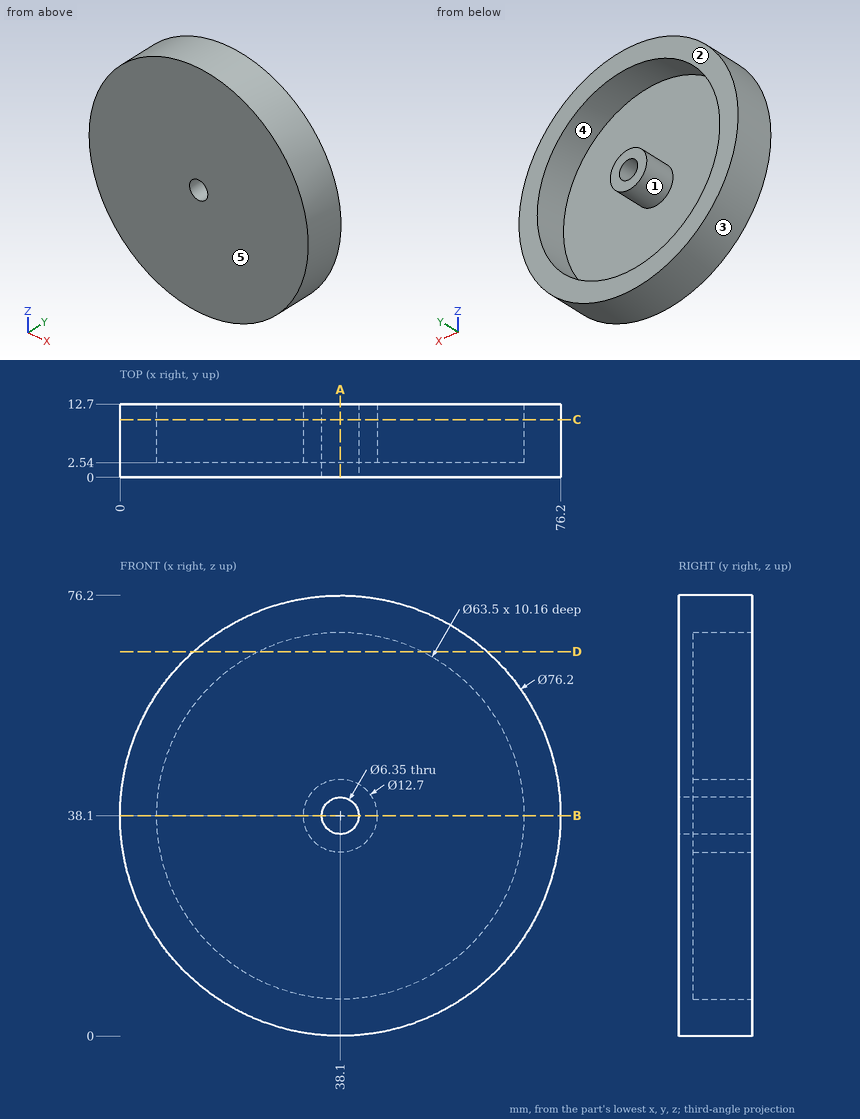
Geometry: see drawing. Coordinates: mm, zero at the bounding-box minimum. A direction names the side the tool comes from. Round coordinates to 2 decimals unless told otherwise and drop trailing zeros. Order: outer loops, then holes, each group sorted by start corner. A loop starts at its lowest first (then second) coordinate and runs counter-clockwise, first axis right, second up. Notation, with made-up numbers: (11.25, -12) - (69.25, -12) arc R23 cw to (69.25, 9) - close; hole circle Ø2 at (48.5, -7). An arc over 180 degrees is marked (long way). One line per question, with ' | ' between items. Start each with the question number.
1) Pull-direction query (X, two-part tool) for the marked faces 3, 4 and 5; classes: +X half, -X half, draft (parallel to the pull), parting line (faces both ways), or undercut.
2) Set-up query: the marked faces 1 and 2. Return all of +Z, -Z, +X, -X, +Y, -Y with unobstructed straight access to the full face (end or side cutting, diameter ignored); none if empty.
3) Contact query for flat-ended pins moving along their axis: P1, Ø2, axis at y = 7.5, z = 64, coming from the -X side; P2, Ø5, axis at x = 9, y = 10, coming from the -Z side; P3, Ø1, axis at x = 21, y = 7.5, coming from the -Z side. Output: stop coordinate, or through.
4) Cut plane A-A, the plane x = 38.1. Return the cut outline in (y, z) (3 decimals), then the cut area to 3 significant figures.
5) Cut plane C-C, the plane y = 10. Return the cut outline in (x, z) (3 decimals).
6) Ray query, probe 1 along Z at (x, y) = (38.1, 9) (3 decimals); probe 2 along Z at (x, y) = (33, 8.25); probe 3 along Y at (x, z) = (59, 52). Return the intervals inside material, ascending.
7) Cut plane D-D, the plane z = 66.5. Return the cut outline in (x, y), then the cut area to 3 significant figures.
8) Cut plane B-B, the plane z = 38.1. Return the cut outline in (x, y) (3 decimals), then the cut area to 3 significant figures.
Worked out:
1) face 3: parting line | face 4: undercut | face 5: draft
2) face 1: +Y | face 2: +Z, -Z, +X, -X, +Y
3) P1: stops at x = 9.26 | P2: stops at z = 10.82 | P3: stops at z = 3.81
4) outline: (0, 0) - (12.7, 0) - (12.7, 6.35) - (2.54, 6.35) - (2.54, 31.75) - (12.7, 31.75) - (12.7, 34.925) - (0, 34.925) - close; (0, 41.275) - (12.7, 41.275) - (12.7, 44.45) - (2.54, 44.45) - (2.54, 69.85) - (12.7, 69.85) - (12.7, 76.2) - (0, 76.2) - close | area: 371 mm^2
5) outline: circle Ø76.2 at (38.1, 38.1); circle Ø12.7 at (38.1, 38.1); hole circle Ø63.5 at (38.1, 38.1); hole circle Ø6.35 at (38.1, 38.1)
6) probe 1: z = 0 to 6.35, 31.75 to 34.925, 41.275 to 44.45, 69.85 to 76.2 | probe 2: z = 0.34 to 6.76, 34.32 to 41.88, 69.44 to 75.86 | probe 3: y = 0 to 2.54
7) outline: (12.7, 0) - (63.5, 0) - (63.5, 12.7) - (52.3, 12.7) - (52.3, 2.54) - (23.9, 2.54) - (23.9, 12.7) - (12.7, 12.7) - close | area: 357 mm^2
8) outline: (0, 0) - (34.925, 0) - (34.925, 12.7) - (31.75, 12.7) - (31.75, 2.54) - (6.35, 2.54) - (6.35, 12.7) - (0, 12.7) - close; (41.275, 0) - (76.2, 0) - (76.2, 12.7) - (69.85, 12.7) - (69.85, 2.54) - (44.45, 2.54) - (44.45, 12.7) - (41.275, 12.7) - close | area: 371 mm^2
